```python
from build123d import *

# Parameters (mm, degrees)
F0_R     = 2.5
F1_DEPTH = 5
F3_DEPTH = 10
F4_SIZE  = 5
F6_R     = 22.558117
F7_DEPTH = 25
F9_DEPTH = 48


with BuildPart() as f1:
    # F0 (on Front) → F1 (new body)
    with BuildSketch(Plane.XZ):
        Circle(F0_R)
    extrude(amount=F1_DEPTH)

    # F2 (on Top) → F3 (join, symmetric)
    with BuildSketch(Plane.XY):
        Polygon((-14.046734, 0), (0, 0), (14.046734, 0), (31.45878, 33.222206), (31.45878, 120), (0, 120), (-31.45878, 120), (-31.45878, 33.222206), align=None)
    extrude(amount=F3_DEPTH, both=True)

    # F4
    f4_edges = [f1.edges().sort_by_distance(p)[0] for p in [
        (-31.45878, 76.611103, -10),
        (-22.752757, 16.611103, -10),
        (0, 0, -10),
        (22.752757, 16.611103, -10),
        (31.45878, 76.611103, -10),
        (31.45878, 76.611103, 10),
        (22.752757, 16.611103, 10),
        (0, 0, 10),
        (-22.752757, 16.611103, 10),
        (-31.45878, 76.611103, 10),
    ]]
    chamfer(f4_edges, length=F4_SIZE)

    # F6 (on offset) → F7 (join)
    with BuildSketch(Plane.XZ.offset(-70)):
        Circle(F6_R)
    extrude(amount=F7_DEPTH)

    # F8 (on offset) → F9 (join)
    with BuildSketch(Plane.XZ.offset(-70)):
        Polygon((26.45878, -97), (26.45878, -10), (0, -10), (-26.45878, -10), (-26.45878, -97), (0, -97), align=None)
    extrude(amount=-F9_DEPTH)


solid = f1.part
```
Work out the finished part from the listing and answer in its coordinate system (mm). A direction names the side the tool comes from. Coordinates: 2 decimals unless noted, no trailing zeros. Write each loop counter-clockwise with the first axis right and the second up, starting at its lowest first coordinate (ties: lowest second). Pieces come first, ordered by that corner, then holes. Notation, with made-up numbers: (9, 78.25) - (29, 78.25) arc R25 cw to (29, 115.25) - close; hole circle Ø10 at (12, -26). An arc over 180 degrees is marked (long way). Answer as a JSON object with one key per item and string values.
Q1. Find section A-A (y = 76). Write down the section's boundary in (x, z).
Results list:
{"outline": "(-31.46, -5) - (-26.46, -10) - (-26.46, -97) - (26.46, -97) - (26.46, -10) - (31.46, -5) - (31.46, 5) - (26.46, 10) - (-26.46, 10) - (-31.46, 5) - close"}
Q2. Given pin 1 Ø14 at (x, z) = (3, -14.5) entering from -Y; pin 2 Ø5 at (y, z) = (50.5, 10) entering from -X; pin 3 Ø5 at (x, z) = (24, 2) entering from -Y, each flat-ended and moving along its own axis, determine where each tip first touches the part or whether it passes through.
Results list:
{"pin 1": "stops at y = 2.5", "pin 2": "stops at x = -28.96", "pin 3": "stops at y = 14.22"}
Q3. Find section B-B (z = 0). Write down the section's boundary in (x, y).
Results list:
{"outline": "(-31.46, 33.22) - (-14.05, 0) - (-2.5, 0) - (-2.5, -5) - (2.5, -5) - (2.5, 0) - (14.05, 0) - (31.46, 33.22) - (31.46, 120) - (-31.46, 120) - close"}
Q4. Consider L1, parallel to Z at x = 18, y = 27; L2, parallel to Z at x = 21.5, y = 92.5; L3, parallel to X at y = 98, z = -12.5. Determine where each line is inside the solid, lowest interval first. Write a range as from..to.
Results list:
{"L1": "z = -10..10", "L2": "z = -97..10", "L3": "x = -26.46..26.46"}
Q5. Find section C-C (x = 0). Write down the section's boundary in (y, z).
Results list:
{"outline": "(-5, -2.5) - (0, -2.5) - (0, -5) - (5, -10) - (45, -10) - (45, -22.56) - (70, -22.56) - (70, -97) - (118, -97) - (118, -10) - (120, -10) - (120, 10) - (70, 10) - (70, 22.56) - (45, 22.56) - (45, 10) - (5, 10) - (0, 5) - (0, 2.5) - (-5, 2.5) - close"}
Q6. Which of the six approach directions +Z, -Z, +X, -X, +Y, -Y give full straight-line access (tool end or side, diameter ignored) to faces 1 (the flat face through (0, 70, 15)), 2 (the flat face through (-26.459, 94, -53)), 3 (the cylindrical face through (-0.54, -2.46, -2.44)), 4 (the flat face through (26.459, 94, -54)), 5 (the cylindrical face through (0.351, 57.675, 22.555))?
Results list:
{"face 1": "+Z, +X, -X, +Y", "face 2": "-Z, -X, +Y, -Y", "face 3": "-Y", "face 4": "-Z, +X, +Y, -Y", "face 5": "+Z, +Y, -Y"}
Q7. Find section D-D (x = -16). Write down the section's boundary in (y, z), plus the area to 3 significant figures.
Results list:
{"outline": "(3.73, -5) - (14.5, -10) - (45, -10) - (45, -15.9) - (70, -15.9) - (70, -97) - (118, -97) - (118, -10) - (120, -10) - (120, 10) - (70, 10) - (70, 15.9) - (45, 15.9) - (45, 10) - (14.5, 10) - (3.73, 5) - close", "area": "6,740 mm^2"}
